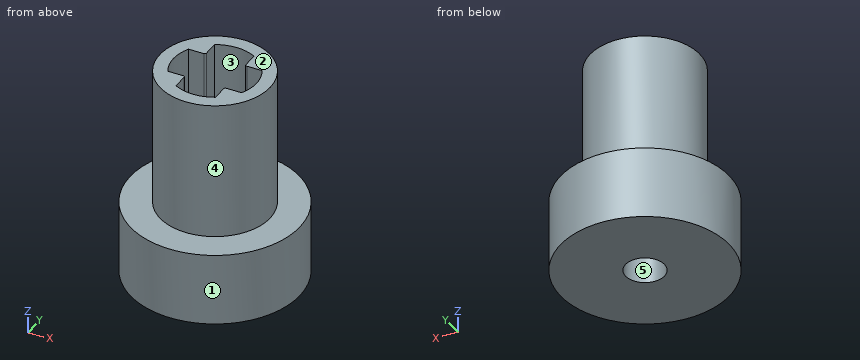
from build123d import *

# Parameters (mm, degrees)
SKETCH_1_R          = 5
SKETCH_1_R_2        = 1.15
EXTRUDE_1_DEPTH     = 12.5
CUT_EXTRUDE_START   = -8.2
SKETCH_2_R          = 5
SKETCH_2_R_2        = 3.25
CUT_EXTRUDE_5_DEPTH = 8.2
CUT_EXTRUDE_START_2 = -8
SKETCH_2_7_R        = 1.15
CUT_EXTRUDE_6_DEPTH = 8
FILLET_1_R          = 0.1


with BuildPart() as part:
    # 草图1 → 凸台-拉伸1 (new body)
    with BuildSketch(Plane.XY):
        Circle(SKETCH_1_R)
        Circle(SKETCH_1_R_2, mode=Mode.SUBTRACT)
    extrude(amount=EXTRUDE_1_DEPTH)

    # 草图2 → 切除-拉伸5 (cut)
    with BuildSketch(Plane.XY.offset(12.5).offset(CUT_EXTRUDE_START)):
        Circle(SKETCH_2_R)
        Circle(SKETCH_2_R_2, mode=Mode.SUBTRACT)
    extrude(amount=CUT_EXTRUDE_5_DEPTH, mode=Mode.SUBTRACT)

    # 草图2<7> → 切除-拉伸6 (cut)
    with BuildSketch(Plane.XY.offset(12.5).offset(CUT_EXTRUDE_START_2)):
        with BuildLine():
            Line((2.158689242, 1.158689242), (1.158689242, 1.158689242))
            Line((1.158689242, 1.158689242), (1.158689242, 2.158689242))
            ThreePointArc((1.158689242, 2.158689242), (0, 2.45), (-1.158689242, 2.158689242))
            Line((-1.158689242, 2.158689242), (-1.158689242, 1.158689242))
            Line((-1.158689242, 1.158689242), (-2.158689242, 1.158689242))
            ThreePointArc((-2.158689242, 1.158689242), (-2.45, 0), (-2.158689242, -1.158689242))
            Line((-2.158689242, -1.158689242), (-1.158689242, -1.158689242))
            Line((-1.158689242, -1.158689242), (-1.158689242, -2.158689242))
            ThreePointArc((-1.158689242, -2.158689242), (0, -2.45), (1.158689242, -2.158689242))
            Line((1.158689242, -2.158689242), (1.158689242, -1.158689242))
            Line((1.158689242, -1.158689242), (2.158689242, -1.158689242))
            ThreePointArc((2.158689242, -1.158689242), (2.376056464, -0.597373986), (2.45, 0))
            ThreePointArc((2.45, 0), (2.376056464, 0.597373986), (2.158689242, 1.158689242))
        make_face()
        Circle(SKETCH_2_7_R, mode=Mode.SUBTRACT)
    extrude(amount=CUT_EXTRUDE_6_DEPTH, mode=Mode.SUBTRACT)

    # 圆角1
    fillet_1_edges = [part.edges().sort_by_distance(p)[0] for p in [
        (1.158689242, 1.158689242, 8.5),
        (1.158689242, -1.158689242, 8.5),
        (-1.158689242, -1.158689242, 8.5),
        (-1.158689242, 1.158689242, 8.5),
    ]]
    fillet(fillet_1_edges, radius=FILLET_1_R)


solid = part.part
Input: part model. Units: mm. Frame: model coordinates. Face numbers are marked on the shaded views. A direction names the side the tool comes from. Round coordinates to 2 decimals unless told otherwise and drop trailing zeros. Order: outer loops, then holes, each group sorted by start corner. A loop starts at its lowest first (then second) coordinate and runs counter-clockwise, first axis right, second up.
1. Pin query (flat end, axial travel): P1, Ø1.5, axis at x = -1, y = -2, coming from the -Z side; P2, Ø0.5, axis at y = -1.5, z = 7, coming from the -X side; P3, Ø0.7, axis at y = -1.5, z = 10, coming from the +X side; P4, Ø1, axis at x = -1.5, z = 8.5, coming from the -Y side. Return the tip coordinate at first contact, or that it passes through.
The answers:
P1: stops at z = 0
P2: stops at x = -3
P3: stops at x = 3.04
P4: stops at y = -3.09
2. Material intervals for line 1 (Y direction, x = 0, z = 1.7); line 2 (Z direction, x = -2.25, y = -0.75); line 3 (Y direction, x = 1.75, z = 11), sorted ascending.
The answers:
line 1: y = -5 to -1.15, 1.15 to 5
line 2: z = 0 to 4.5
line 3: y = -2.74 to -1.16, 1.16 to 2.74
3. Cut plane A-A, the plane x = 0. Output: boundary loops of the cut face in (y, z), then the cut area to 4 significant figures.
The answers:
outline: (-5, 0) - (-1.15, 0) - (-1.15, 4.5) - (-2.45, 4.5) - (-2.45, 12.5) - (-3.25, 12.5) - (-3.25, 4.3) - (-5, 4.3) - close; (1.15, 0) - (5, 0) - (5, 4.3) - (3.25, 4.3) - (3.25, 12.5) - (2.45, 12.5) - (2.45, 4.5) - (1.15, 4.5) - close
area: 46.75 mm2
4. Cut plane B-B, the plane y = -0.25. Output: boundary loops of the cut face in (x, z).
The answers:
outline: (-4.99, 0) - (-1.12, 0) - (-1.12, 4.5) - (-2.44, 4.5) - (-2.44, 12.5) - (-3.24, 12.5) - (-3.24, 4.3) - (-4.99, 4.3) - close; (1.12, 0) - (4.99, 0) - (4.99, 4.3) - (3.24, 4.3) - (3.24, 12.5) - (2.44, 12.5) - (2.44, 4.5) - (1.12, 4.5) - close
5. Cut plane C-C, the plane z = 11.25. Output: boundary loops of the cut face in (x, y).
The answers:
outline: circle Ø6.5 at (0, 0); hole (-2.16, -1.16) - (-1.26, -1.16) arc R0.1 cw to (-1.16, -1.26) - (-1.16, -2.16) arc R2.45 ccw to (1.16, -2.16) - (1.16, -1.26) arc R0.1 cw to (1.26, -1.16) - (2.16, -1.16) arc R2.45 ccw to (2.16, 1.16) - (1.26, 1.16) arc R0.1 cw to (1.16, 1.26) - (1.16, 2.16) arc R2.45 ccw to (-1.16, 2.16) - (-1.16, 1.26) arc R0.1 cw to (-1.26, 1.16) - (-2.16, 1.16) arc R2.45 ccw to start
6. Mould query, pull axis X, two halves, no side actions, for the marked faces 1, 2 and 3. Classes: released by +X, released by -X, zero draft, split by the parting line, or undercut.
The answers:
face 1: split by the parting line
face 2: zero draft
face 3: undercut
7. Cut plane D-D, the plane y = 3. Output: boundary loops of the cut face in (x, z).
The answers:
outline: (-4, 0) - (4, 0) - (4, 4.3) - (1.25, 4.3) - (1.25, 12.5) - (-1.25, 12.5) - (-1.25, 4.3) - (-4, 4.3) - close
8. Set-up query: the marked faces 4 and 5. Return all of +Z, -Z, +X, -X, +Y, -Y with unobstructed straight access to the full face (end or side cutting, diameter ignored); none if empty.
The answers:
face 4: +Z
face 5: +Z, -Z
